Read the model definition and answer for the solid it produces. Units are mm, in the model's axes. A direction names the side the tool comes from. Round coordinates to 2 decimals unless told otherwise and drop trailing zeros. Order: outer loops, then holes, each group sorted by start corner. A loop starts at its lowest first (then second) coordinate and runs counter-clockwise, first axis right, second up. Notation, with made-up numbers: (77, 43) -> (86, 43) arc R19 cw to (86, 56) -> close; hole circle Ø9 at (48, 37.25). An arc over 180 degrees is marked (long way). Answer as a JSON object with one key per item and string values. Group by question number.
Item 1: Section C-C, the plane x = -8.5 is taken. Write down the section's boundary in (y, z), plus the area to 3 significant figures.
Item 2: For faces 4 (the cylindrical face through (-10.006, 11.86, -2.222)), 5 (the flat face through (0, -10, 3)), 6 (the cylindrical face through (-3.905, -4.93, 0.867)), determine the directions among +Z, -Z, +X, -X, +Y, -Y from which every point of the face is accessible in a straight line to the end or side of a thin tool.
Item 3: Section A-A, the plane y = -2 is taken. Write down the section's boundary in (x, z), plus the area to 3 significant figures.
Item 4: Given P1, Ø1.5, axis at y = 4, z = 10, coming from the -X side; P2, Ø5, axis at x = -9.5, y = 1.5, coming from the +Z side; P3, Ø3, axis at y = 5, z = -11, coming from the +X side, each flat-ended and moving along its own axis, determine where each tip first touches the part or whether it passes through.
Item 5: Consider probe 1 along Y at (x, z) = (-14, 3); probe 2 along Y at (x, z) = (5.5, -8.5); probe 3 along Z at (x, y) = (2, -2.5). Determine where each line is inside the solid, lowest interval first. Write a range as from..to.
Item 6: Section D-D, the plane y = 18.5 is taken. Write down the section's boundary in (x, z), plus the area to 3 significant figures.
Item 7: The mould has two halves that part along Z. Classify faces 1 (the flat face through (0, 6, 2.485)), 2 (the flat face through (2.4, 22, -2.4)), 3 (the cylindrical face through (-15.62, 0.99, -3.47)): pulls with the +Z half, pulls with the -Z half, needs draft (parallel to the pull), parting line crosses it, or undercut.
Item 8: Section B-B, the plane z = 8.5 is taken. Write down the section's boundary in (x, y), plus the area to 3 significant figures.
from build123d import *

# Parameters (mm, degrees)
SKETCH1_R               = 16
BOSS_EXTRUDE1_DEPTH     = 2
SKETCH2_R               = 10.25
BOSS_EXTRUDE2_DEPTH     = 20
SKETCH4_R               = 4
BOSS_EXTRUDE3_DEPTH     = 10
CUT_EXTRUDE1_DEPTH      = 32.559467676
CUT_EXTRUDE1_DEPTH_BACK = 32.559467676


with BuildPart() as part:
    # Sketch1 → Boss-Extrude1 (new body)
    with BuildSketch(Plane(origin=(0, 0, 0), x_dir=(1, 0, 0), z_dir=(0, 1, 0))):
        with Locations(Location((0, 0, 0), (0, 0, 270))):
            Circle(SKETCH1_R)
    extrude(amount=BOSS_EXTRUDE1_DEPTH)

    # Sketch2 → Boss-Extrude2 (add)
    with BuildSketch(Plane(origin=(0, 2, 0), x_dir=(1, 0, 0), z_dir=(0, 1, 0))):
        with Locations(Location((0, 0, 0), (0, 0, 270))):
            Circle(SKETCH2_R)
    extrude(amount=BOSS_EXTRUDE2_DEPTH)

    # Sketch4 → Boss-Extrude3 (add)
    with BuildSketch(Plane.XZ):
        with Locations(Location((0, 0, 0), (0, 0, 270))):
            Circle(SKETCH4_R)
    extrude(amount=BOSS_EXTRUDE3_DEPTH)

    # Sketch3 → Cut-Extrude1 (cut, two sides: drawn at the far end of the back side and taken through both)
    with BuildSketch(Plane.XZ.offset(-CUT_EXTRUDE1_DEPTH_BACK)):
        with BuildLine():
            Line((0, 2.484658643), (0, -3.1))
            ThreePointArc((0, -3.1), (2.192031022, -2.192031022), (3.1, 0))
            ThreePointArc((3.1, 0), (2.770983027, 1.389839223), (1.853772215, 2.484658643))
            Line((1.853772215, 2.484658643), (0, 2.484658643))
        make_face()
        with BuildLine():
            ThreePointArc((-1.853772215, 2.484658643), (-2.942145628, -0.976616149), (0, -3.1))
            Line((0, -3.1), (0, 2.484658643))
            Line((0, 2.484658643), (-1.853772215, 2.484658643))
        make_face()
    extrude(amount=CUT_EXTRUDE1_DEPTH + CUT_EXTRUDE1_DEPTH_BACK, mode=Mode.SUBTRACT)


solid = part.part
Values found:
{
 "1": {"outline": "(0, -13.56) -> (2, -13.56) -> (2, -5.73) -> (22, -5.73) -> (22, 5.73) -> (2, 5.73) -> (2, 13.56) -> (0, 13.56) -> close", "area": "283 mm2"},
 "2": {"face 4": "+Y", "face 5": "+Z, -Z, +X, -X, -Y", "face 6": "-Y"},
 "3": {"outline": "circle Ø8 at (0, 0); hole (-1.85, 2.48) arc R3.1 ccw (long way) to (1.85, 2.48) -> close", "area": "21.6 mm2"},
 "4": {"P1": "x = -4.42", "P2": "z = 14.39", "P3": "x = 3.85"},
 "5": {"probe 1": "0..2", "probe 2": "0..22", "probe 3": "-3.46..-2.37, 2.37..3.46"},
 "6": {"outline": "circle Ø20.5 at (0, 0); hole (-1.85, 2.48) arc R3.1 ccw (long way) to (1.85, 2.48) -> close", "area": "301 mm2"},
 "7": {"face 1": "undercut", "face 2": "needs draft", "face 3": "parting line crosses it"},
 "8": {"outline": "(-13.56, 0) -> (13.56, 0) -> (13.56, 2) -> (5.73, 2) -> (5.73, 22) -> (-5.73, 22) -> (-5.73, 2) -> (-13.56, 2) -> close", "area": "283 mm2"}
}
